Verification items for the finished model (mm, model axes). Give positions to 0.01 mm unless a question says otherwise; leave off trailing zeros. Loops run counter-clockwise (first coordinate to the right, second up) from the corner with the lowest first, then second, coordinate; pieces in that order, holes last. Notation, with made-up numbers: (-32.5, -11) - (8.5, -11) arc R19 ccw to (8.5, -3) - close; hole circle Ø9 at (64, 18.25). An arc over 180 degrees is marked (long way). Use one line per item in the form item = value.
```python
from build123d import *

# Parameters (mm, degrees)
ESQUISSE1_W             = 196
ESQUISSE1_H             = 55
BOSS_EXTRU_1_DEPTH      = 1.5
CONG_1_R                = 4
ESQUISSE2_R             = 2
ENL_V_MAT_EXTRU_1_DEPTH = 102.796365358
ENL_V_MAT_EXTRU_2_REACH = 103.796
ESQUISSE3_R             = 1.6
ENL_V_MAT_EXTRU_3_REACH = 103.796
ESQUISSE4_R             = 1.6


with BuildPart() as part:
    # Esquisse1 → Boss.-Extru.1 (new body)
    with BuildSketch(Plane.XY):
        Rectangle(ESQUISSE1_W, ESQUISSE1_H)
    extrude(amount=BOSS_EXTRU_1_DEPTH)

    # Congé1
    cong_1_edges = [part.edges().sort_by_distance(p)[0] for p in [
        (-98, 27.5, 0.75),
        (98, 27.5, 0.75),
        (98, -27.5, 0.75),
        (-98, -27.5, 0.75),
    ]]
    fillet(cong_1_edges, radius=CONG_1_R)

    # Esquisse2 → Enlèv. mat.-Extru.1 (cut, through all)
    with BuildSketch(Plane.XY.offset(1.5)):
        with Locations((-90, 19.5)):
            Circle(ESQUISSE2_R)
        with Locations((-90, -19.5)):
            Circle(ESQUISSE2_R)
        with Locations((90, 19.5)):
            Circle(ESQUISSE2_R)
        with Locations((90, -19.5)):
            Circle(ESQUISSE2_R)
    extrude(amount=-ENL_V_MAT_EXTRU_1_DEPTH, mode=Mode.SUBTRACT)

    # Esquisse3 → Enlèv. mat.-Extru.2 (cut, up to next)
    with BuildSketch(Plane.XY.offset(1.5), mode=Mode.PRIVATE) as enl_v_mat_extru_2_sk1:
        with Locations((-51.2, 24)):
            Circle(ESQUISSE3_R)
    enl_v_mat_extru_2_tool1 = extrude(enl_v_mat_extru_2_sk1.sketch, amount=-ENL_V_MAT_EXTRU_2_REACH, mode=Mode.PRIVATE) & part.part
    # Esquisse3 → Enlèv. mat.-Extru.2 (cut, up to next)
    with BuildSketch(Plane.XY.offset(1.5), mode=Mode.PRIVATE) as enl_v_mat_extru_2_sk2:
        with Locations((-40.2, 24)):
            Circle(ESQUISSE3_R)
    enl_v_mat_extru_2_tool2 = extrude(enl_v_mat_extru_2_sk2.sketch, amount=-ENL_V_MAT_EXTRU_2_REACH, mode=Mode.PRIVATE) & part.part
    # Esquisse3 → Enlèv. mat.-Extru.2 (cut, up to next)
    with BuildSketch(Plane.XY.offset(1.5), mode=Mode.PRIVATE) as enl_v_mat_extru_2_sk3:
        with Locations((-40.2, -24)):
            Circle(ESQUISSE3_R)
    enl_v_mat_extru_2_tool3 = extrude(enl_v_mat_extru_2_sk3.sketch, amount=-ENL_V_MAT_EXTRU_2_REACH, mode=Mode.PRIVATE) & part.part
    # Esquisse3 → Enlèv. mat.-Extru.2 (cut, up to next)
    with BuildSketch(Plane.XY.offset(1.5), mode=Mode.PRIVATE) as enl_v_mat_extru_2_sk4:
        with Locations((-51.2, -24)):
            Circle(ESQUISSE3_R)
    enl_v_mat_extru_2_tool4 = extrude(enl_v_mat_extru_2_sk4.sketch, amount=-ENL_V_MAT_EXTRU_2_REACH, mode=Mode.PRIVATE) & part.part
    # Esquisse3 → Enlèv. mat.-Extru.2 (cut, up to next)
    with BuildSketch(Plane.XY.offset(1.5), mode=Mode.PRIVATE) as enl_v_mat_extru_2_sk5:
        with Locations((40.2, -24)):
            Circle(ESQUISSE3_R)
    enl_v_mat_extru_2_tool5 = extrude(enl_v_mat_extru_2_sk5.sketch, amount=-ENL_V_MAT_EXTRU_2_REACH, mode=Mode.PRIVATE) & part.part
    # Esquisse3 → Enlèv. mat.-Extru.2 (cut, up to next)
    with BuildSketch(Plane.XY.offset(1.5), mode=Mode.PRIVATE) as enl_v_mat_extru_2_sk6:
        with Locations((51.2, -24)):
            Circle(ESQUISSE3_R)
    enl_v_mat_extru_2_tool6 = extrude(enl_v_mat_extru_2_sk6.sketch, amount=-ENL_V_MAT_EXTRU_2_REACH, mode=Mode.PRIVATE) & part.part
    # Esquisse3 → Enlèv. mat.-Extru.2 (cut, up to next)
    with BuildSketch(Plane.XY.offset(1.5), mode=Mode.PRIVATE) as enl_v_mat_extru_2_sk7:
        with Locations((51.2, 24)):
            Circle(ESQUISSE3_R)
    enl_v_mat_extru_2_tool7 = extrude(enl_v_mat_extru_2_sk7.sketch, amount=-ENL_V_MAT_EXTRU_2_REACH, mode=Mode.PRIVATE) & part.part
    # Esquisse3 → Enlèv. mat.-Extru.2 (cut, up to next)
    with BuildSketch(Plane.XY.offset(1.5), mode=Mode.PRIVATE) as enl_v_mat_extru_2_sk8:
        with Locations((40.2, 24)):
            Circle(ESQUISSE3_R)
    enl_v_mat_extru_2_tool8 = extrude(enl_v_mat_extru_2_sk8.sketch, amount=-ENL_V_MAT_EXTRU_2_REACH, mode=Mode.PRIVATE) & part.part
    add(enl_v_mat_extru_2_tool1.solids().sort_by_distance((-51.2, 24, 1.5))[0], mode=Mode.SUBTRACT)
    add(enl_v_mat_extru_2_tool2.solids().sort_by_distance((-40.2, 24, 1.5))[0], mode=Mode.SUBTRACT)
    add(enl_v_mat_extru_2_tool3.solids().sort_by_distance((-40.2, -24, 1.5))[0], mode=Mode.SUBTRACT)
    add(enl_v_mat_extru_2_tool4.solids().sort_by_distance((-51.2, -24, 1.5))[0], mode=Mode.SUBTRACT)
    add(enl_v_mat_extru_2_tool5.solids().sort_by_distance((40.2, -24, 1.5))[0], mode=Mode.SUBTRACT)
    add(enl_v_mat_extru_2_tool6.solids().sort_by_distance((51.2, -24, 1.5))[0], mode=Mode.SUBTRACT)
    add(enl_v_mat_extru_2_tool7.solids().sort_by_distance((51.2, 24, 1.5))[0], mode=Mode.SUBTRACT)
    add(enl_v_mat_extru_2_tool8.solids().sort_by_distance((40.2, 24, 1.5))[0], mode=Mode.SUBTRACT)

    # Esquisse4 → Enlèv. mat.-Extru.3 (cut, up to next)
    with BuildSketch(Plane.XY.offset(1.5), mode=Mode.PRIVATE) as enl_v_mat_extru_3_sk1:
        with Locations((-70, 24)):
            Circle(ESQUISSE4_R)
    enl_v_mat_extru_3_tool1 = extrude(enl_v_mat_extru_3_sk1.sketch, amount=-ENL_V_MAT_EXTRU_3_REACH, mode=Mode.PRIVATE) & part.part
    # Esquisse4 → Enlèv. mat.-Extru.3 (cut, up to next)
    with BuildSketch(Plane.XY.offset(1.5), mode=Mode.PRIVATE) as enl_v_mat_extru_3_sk2:
        with Locations((0, 24)):
            Circle(ESQUISSE4_R)
    enl_v_mat_extru_3_tool2 = extrude(enl_v_mat_extru_3_sk2.sketch, amount=-ENL_V_MAT_EXTRU_3_REACH, mode=Mode.PRIVATE) & part.part
    # Esquisse4 → Enlèv. mat.-Extru.3 (cut, up to next)
    with BuildSketch(Plane.XY.offset(1.5), mode=Mode.PRIVATE) as enl_v_mat_extru_3_sk3:
        with Locations((70, 24)):
            Circle(ESQUISSE4_R)
    enl_v_mat_extru_3_tool3 = extrude(enl_v_mat_extru_3_sk3.sketch, amount=-ENL_V_MAT_EXTRU_3_REACH, mode=Mode.PRIVATE) & part.part
    # Esquisse4 → Enlèv. mat.-Extru.3 (cut, up to next)
    with BuildSketch(Plane.XY.offset(1.5), mode=Mode.PRIVATE) as enl_v_mat_extru_3_sk4:
        with Locations((70, -24)):
            Circle(ESQUISSE4_R)
    enl_v_mat_extru_3_tool4 = extrude(enl_v_mat_extru_3_sk4.sketch, amount=-ENL_V_MAT_EXTRU_3_REACH, mode=Mode.PRIVATE) & part.part
    # Esquisse4 → Enlèv. mat.-Extru.3 (cut, up to next)
    with BuildSketch(Plane.XY.offset(1.5), mode=Mode.PRIVATE) as enl_v_mat_extru_3_sk5:
        with Locations((0, -24)):
            Circle(ESQUISSE4_R)
    enl_v_mat_extru_3_tool5 = extrude(enl_v_mat_extru_3_sk5.sketch, amount=-ENL_V_MAT_EXTRU_3_REACH, mode=Mode.PRIVATE) & part.part
    # Esquisse4 → Enlèv. mat.-Extru.3 (cut, up to next)
    with BuildSketch(Plane.XY.offset(1.5), mode=Mode.PRIVATE) as enl_v_mat_extru_3_sk6:
        with Locations((-70, -24)):
            Circle(ESQUISSE4_R)
    enl_v_mat_extru_3_tool6 = extrude(enl_v_mat_extru_3_sk6.sketch, amount=-ENL_V_MAT_EXTRU_3_REACH, mode=Mode.PRIVATE) & part.part
    add(enl_v_mat_extru_3_tool1.solids().sort_by_distance((-70, 24, 1.5))[0], mode=Mode.SUBTRACT)
    add(enl_v_mat_extru_3_tool2.solids().sort_by_distance((0, 24, 1.5))[0], mode=Mode.SUBTRACT)
    add(enl_v_mat_extru_3_tool3.solids().sort_by_distance((70, 24, 1.5))[0], mode=Mode.SUBTRACT)
    add(enl_v_mat_extru_3_tool4.solids().sort_by_distance((70, -24, 1.5))[0], mode=Mode.SUBTRACT)
    add(enl_v_mat_extru_3_tool5.solids().sort_by_distance((0, -24, 1.5))[0], mode=Mode.SUBTRACT)
    add(enl_v_mat_extru_3_tool6.solids().sort_by_distance((-70, -24, 1.5))[0], mode=Mode.SUBTRACT)


solid = part.part
```
1. Scan lines: probe 1 along Y at (x, z) = (40.2, 1); probe 2 along Y at (x, z) = (90, 0.5). Record each from-to range of solid material in increasing order.
Result set:
probe_1 = -27.5 to -25.6, -22.4 to 22.4, 25.6 to 27.5
probe_2 = -27.5 to -21.5, -17.5 to 17.5, 21.5 to 27.5
2. Draft check along X on faces 1 (the cylindrical face through (91.908, 20.101, 0.76)), 2 (the flat face through (-1, 0, 1.5)), 3 (the cylindrical face through (91.908, -18.899, 0.76)), 4 (the cylindrical face through (96.859, 26.297, 0.76)). Enter one of: released by +X, released by -X, zero draft, split by the parting line, or undercut.
Result set:
face_1 = undercut
face_2 = zero draft
face_3 = undercut
face_4 = released by +X
3. Section check A-A, the plane x = -90. Record the cut outline in (y, z), then the cut area to 3 significant figures.
Result set:
outline = (-27.5, 0) - (-21.5, 0) - (-21.5, 1.5) - (-27.5, 1.5) - close; (-17.5, 0) - (17.5, 0) - (17.5, 1.5) - (-17.5, 1.5) - close; (21.5, 0) - (27.5, 0) - (27.5, 1.5) - (21.5, 1.5) - close
area = 70.5 mm²
4. Section check B-B, the plane z = 0.6. State how many separate pieces and enclosed holes the cut face has, then the cut area to 3 significant figures.
Result set:
separate_pieces = 1
enclosed_holes = 18
area = 10,600 mm²
